```python
from build123d import *

# Parameters (mm, degrees)
SKETCH1_R           = 1.869394483
SKETCH1_R_2         = 1.6775
SKETCH1_R_3         = 1.75
SKETCH1_W           = 21.327694626
SKETCH1_H           = 41.102200046
BOSS_EXTRUDE1_DEPTH = 3.8


with BuildPart() as part:
    # Sketch1 → Boss-Extrude1 (new body)
    with BuildSketch(Plane.XY):
        with BuildLine():
            Line((8.585, -14.879916086), (10.629231235, -14.879916086))
            add(Edge.make_bspline(
                [(10.629231235, -14.879916086), (14.945689429, -19.598266914), (11.330822281, -32.912320887), (19.835, -32.631980139)],
                knots=[0, 0, 0, 0, 1, 1, 1, 1], degree=3))
            add(Edge.make_bspline(
                [(29.040768765, -14.879916086), (24.724310571, -19.598266914), (28.339177719, -32.912320887), (19.835, -32.631980139)],
                knots=[0, 0, 0, 0, 1, 1, 1, 1], degree=3))
            Line((29.040768765, -14.879916086), (31.085, -14.879916086))
            ThreePointArc((31.085, -14.879916086), (32.499213562, -14.294129648), (33.085, -12.879916086))
            Line((33.085, -12.879916086), (33.085, 77.107681283))
            ThreePointArc((33.085, 77.107681283), (32.484733836, 78.556851998), (31.035563121, 79.157118162))
            Line((31.035563121, 79.157118162), (8.634436879, 79.157118162))
            ThreePointArc((8.634436879, 79.157118162), (7.185266164, 78.556851998), (6.585, 77.107681283))
            Line((6.585, 77.107681283), (6.585, -12.879916086))
            ThreePointArc((6.585, -12.879916086), (7.170786438, -14.294129648), (8.585, -14.879916086))
        make_face()
        with Locations(Location((19.835, -29.181539917, 0), (0, 0, 180))):
            Circle(SKETCH1_R, mode=Mode.SUBTRACT)
        with Locations(Location((12.335, 9, 0), (0, 0, 180))):
            Circle(SKETCH1_R_2, mode=Mode.SUBTRACT)
        with Locations(Location((12.335, -11, 0), (0, 0, 180))):
            Circle(SKETCH1_R_2, mode=Mode.SUBTRACT)
        with Locations(Location((27.335, 9, 0), (0, 0, 180))):
            Circle(SKETCH1_R_2, mode=Mode.SUBTRACT)
        with Locations(Location((27.335, -11, 0), (0, 0, 180))):
            Circle(SKETCH1_R_2, mode=Mode.SUBTRACT)
        with Locations(Location((26.035, 69.924718691, 0), (0, 0, 180))):
            Circle(SKETCH1_R_3, mode=Mode.SUBTRACT)
        with Locations(Location((13.635, 69.924718691, 0), (0, 0, 180))):
            Circle(SKETCH1_R_3, mode=Mode.SUBTRACT)
        with Locations(Location((13.635, 19.524718691, 0), (0, 0, 180))):
            Circle(SKETCH1_R_3, mode=Mode.SUBTRACT)
        with Locations(Location((26.035, 19.524718691, 0), (0, 0, 180))):
            Circle(SKETCH1_R_3, mode=Mode.SUBTRACT)
        with Locations((19.835, 44.774489529)):
            Rectangle(SKETCH1_W, SKETCH1_H, mode=Mode.SUBTRACT)
    extrude(amount=BOSS_EXTRUDE1_DEPTH)


solid = part.part
```
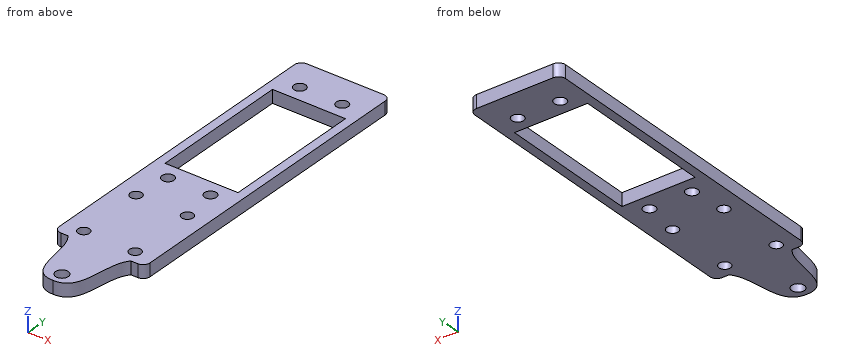
The listing builds one solid part. Answer for the finished solid, in the listing's coordinates (mm). Coordinates: 2 decimals unless noted, no trailing zeros. Loops run counter-clockwise (first coordinate to the right, second up) from the corner with the lowest first, then second, coordinate; pieces in that order, holes last. Notation, with made-up numbers: M 40,56 L 63,56 A31 cw 63,85 Z; hole C 39,86.5 d3. An arc over 180 degrees is marked long. Answer as a JSON object with one key per item and string values. Group by question number.
Item 1: Section C-C (z = 1) is taken. Give the number of separate pieces and of enclosed holes in the cut face, and give its area (3 significant figures).
Item 2: Each of these flat-tipped pins is pushed along its axis until it touches: P1, Ø3, axis at x = 13.64, y = 69.92, coming from the +Z side; P2, Ø1.9, axis at x = 15.5, z = 1, coming from the -Y side; P3, Ø1.5, axis at x = 30, z = 3.5, coming from the -Y side. Where does it stop, or does it pass through?
Item 3: Section B-B (y = -11) is taken. Write down the section's boundary in (x, z) (1 decimal).
Item 4: Section A-A (y = 58) is taken. Write down the section's boundary in (x, z) (3 decimals), and give its area (3 significant figures).
Item 5: Consider L1, parallel to X at y = -11, z = 0.9 (1 decimal); L2, parallel to X at y = 40, z = 2.85 (3 decimals); L3, parallel to X at y = -11.5, z = 0.25 (3 decimals). Determine where each line is inside the solid, lowest interval first.
Solved:
{
 "1": {"separate pieces": "1", "enclosed holes": "10", "area": "1,750 mm2"},
 "2": {"P1": "passes through", "P2": "stops at y = -31.71", "P3": "stops at y = -14.88"},
 "3": {"outline": "M 6.6,0 L 10.7,0 L 10.7,3.8 L 6.6,3.8 Z; M 14,0 L 25.7,0 L 25.7,3.8 L 14,3.8 Z; M 29,0 L 33.1,0 L 33.1,3.8 L 29,3.8 Z"},
 "4": {"outline": "M 6.585,0 L 9.171,0 L 9.171,3.8 L 6.585,3.8 Z; M 30.499,0 L 33.085,0 L 33.085,3.8 L 30.499,3.8 Z", "area": "19.7 mm2"},
 "5": {"L1": "x = 6.6 to 10.7, 14 to 25.7, 29 to 33.1", "L2": "x = 6.585 to 9.171, 30.499 to 33.085", "L3": "x = 6.585 to 10.734, 13.936 to 25.734, 28.936 to 33.085"}
}
